Here's how the part is built. I have some questions about the finished solid (model axes, mm). A direction names the side the tool comes from. Give positions to 0.01 mm unless a question says otherwise; leave off trailing zeros. Write each loop counter-clockwise with the first axis right and the second up, starting at its lowest first coordinate (ties: lowest second). Pieces come first, ordered by that corner, then holes. Notation, with made-up numbers: (-4.5, -18.5) - (30.5, -18.5) arc R21 ccw to (30.5, 3.5) - close; hole circle Ø7 at (50, 42.25). An arc over 180 degrees is marked (long way). Use a Markdown table: item, result.
```python
from build123d import *

# Parameters (mm, degrees)
BOSS_EXTRUDE1_DEPTH    = 3
SKETCH2_R              = 1.625
CUT_EXTRUDE1_DEPTH     = 13.854960132
SKETCH3_R              = 1.625
CUT_EXTRUDE2_DEPTH     = 16.215124055
CONVERT_SOLID1_START   = -3
CONVERT_SOLID1_DEPTH   = 6
CONVERT_SOLID1_2_DEPTH = 6


# Read off the part's stored shape, not the designer's step: Convert-Solid1
with BuildPart() as part:
    # Sketch1 → Boss-Extrude1 (new, symmetric)
    with BuildSketch(Plane(origin=(0, 0, 0), x_dir=(0, 0, -1), z_dir=(1, 0, 0))):
        Polygon((0, 3.5), (0, 0), (9, 0), (9, 1.5), (1.5, 1.5), (1.5, 5), (-13.5, 5), (-13.5, 3.5), align=None)
    extrude(amount=BOSS_EXTRUDE1_DEPTH, both=True)

    # Sketch2 → Cut-Extrude1 (cut, through all)
    with BuildSketch(Plane(origin=(0, 1.5, 1.5), x_dir=(1, 0, 0), z_dir=(0, 1, 0))):
        with Locations(Location((0, 6.5, 0), (0, 0, 270))):
            Circle(SKETCH2_R)
    extrude(amount=-CUT_EXTRUDE1_DEPTH, mode=Mode.SUBTRACT)

    # Sketch3 → Cut-Extrude2 (cut, through all)
    with BuildSketch(Plane(origin=(0, 3.5, -1), x_dir=(1, 0, 0), z_dir=(0, -1, 0))):
        with Locations(Location((0, 10, 0), (0, 0, 270))):
            Circle(SKETCH3_R)
    extrude(amount=-CUT_EXTRUDE2_DEPTH, mode=Mode.SUBTRACT)

    # Convert-Solid1 outline → Convert-Solid1 (cut)
    with BuildSketch(Plane.YZ.offset(CONVERT_SOLID1_START)):
        with BuildLine():
            ThreePointArc((0, -2.25), (0.659009742, -0.659009742), (2.25, 0))
            Line((2.25, 0), (0, 0))
            Line((0, 0), (0, -2.25))
        make_face()
        with BuildLine():
            ThreePointArc((5, 0.75), (4.340990258, -0.840990258), (2.75, -1.5))
            Line((2.75, -1.5), (5, -1.5))
            Line((5, -1.5), (5, 0.75))
        make_face()
    extrude(amount=CONVERT_SOLID1_DEPTH, mode=Mode.SUBTRACT)

    # Convert-Solid1 2 outline → Convert-Solid1 2 (add)
    with BuildSketch(Plane.YZ.offset(CONVERT_SOLID1_START)):
        with BuildLine():
            ThreePointArc((3.5, 0.75), (3.280330086, 0.219669914), (2.75, 0))
            Line((2.75, 0), (3.5, 0))
            Line((3.5, 0), (3.5, 0.75))
        make_face()
        with BuildLine():
            ThreePointArc((1.5, -2.25), (1.719669914, -1.719669914), (2.25, -1.5))
            Line((2.25, -1.5), (1.5, -1.5))
            Line((1.5, -1.5), (1.5, -2.25))
        make_face()
    extrude(amount=CONVERT_SOLID1_2_DEPTH)


solid = part.part
```
Item 1: For faces 1 (the flat face through (0, 3.5, 7)), 2 (the flat face through (0, 4, 13.5)), 3 (the flat face through (0, 1.5, -7)), which set-ups out of +Z, -Z, +X, -X, +Y, -Y let a thin tool reach every point of the face, with its end or its side?
Values:
| item | result |
|---|---|
| face 1 | +Z, +X, -X, -Y |
| face 2 | +Z, +X, -X, +Y, -Y |
| face 3 | -Z, +X, -X, +Y |
Item 2: I need wall thicknesses on line 1 along Y through (x, z) = (1.9, 9); line 2 along X through (y, z) = (4.35, 9) (3 decimals); line 3 along Y through (x, z) = (1.5, -7.75). Which ranges of each line are inside material? Lowest first, please. Write a range as [from, to].
Values:
| item | result |
|---|---|
| line 1 | y = [3.5, 5] |
| line 2 | x = [-3, -1.625], [1.625, 3] |
| line 3 | y = [0, 1.5] |
Item 3: Thinking about a two-plate mould opening in X: for faces 4 (the cylindrical face through (0.071, 4.24, 10.623)), 5 (the flat face through (-3, 4, 2)), 6 (the flat face through (0, 0, -7)), which applies, +X half, -X half, draft (parallel to the pull), parting line (faces both ways), or undercut?
Values:
| item | result |
|---|---|
| face 4 | undercut |
| face 5 | -X half |
| face 6 | draft |
Item 4: If we section it at B-B, the plane x = 0: Write out the boundary of the cut face in (y, z) (3 decimals), plus the area to 3 significant figures.
Values:
| item | result |
|---|---|
| outline | (0, -9) - (1.5, -9) - (1.5, -6.625) - (0, -6.625) - close; (0, -3.375) - (1.5, -3.375) - (1.5, -2.25) arc R0.75 cw to (2.25, -1.5) - (2.75, -1.5) arc R2.25 ccw to (5, 0.75) - (5, 7.375) - (3.5, 7.375) - (3.5, 0.75) arc R0.75 cw to (2.75, 0) - (2.25, 0) arc R2.25 ccw to (0, -2.25) - close; (3.5, 10.625) - (5, 10.625) - (5, 13.5) - (3.5, 13.5) - close |
| area | 27.3 mm2 |
Item 5: If we section it at C-C, the plane y = 4.1: Write out the boundary of the cut face in (x, z) (3 decimals), plus the area to 3 significant figures.
Values:
| item | result |
|---|---|
| outline | (-3, -1.05) - (3, -1.05) - (3, 13.5) - (-3, 13.5) - close; hole circle Ø3.25 at (0, 9) |
| area | 79.0 mm2 |
Item 6: Will these pins go through, and if not, where does the flat tip stop? pin 1 Ø0.6 at (x, y) = (-0.5, 2.5) entering from -Z; pin 2 Ø3.5 at (x, z) = (0, -5) entering from -Y; pin 3 Ø1.9 at (x, z) = (0, 9) entering from +Y; pin 4 Ø3 at (x, z) = (-0.5, 9) entering from -Y.
Values:
| item | result |
|---|---|
| pin 1 | stops at z = -1.5 |
| pin 2 | stops at y = 0 |
| pin 3 | passes through |
| pin 4 | stops at y = 3.5 |
Item 7: If we section it at A-A, the plane z = -5: Write out the boundary of the cut face in (x, y) (3 decimals).
Values:
| item | result |
|---|---|
| outline | (-3, 0) - (-1.625, 0) - (-1.625, 1.5) - (-3, 1.5) - close; (1.625, 0) - (3, 0) - (3, 1.5) - (1.625, 1.5) - close |
Item 8: If we section it at D-D, the plane x = 2.2: Write out the boundary of the cut face in (y, z), plus the area to 3 significant figures.
Values:
| item | result |
|---|---|
| outline | (0, -9) - (1.5, -9) - (1.5, -2.25) arc R0.75 cw to (2.25, -1.5) - (2.75, -1.5) arc R2.25 ccw to (5, 0.75) - (5, 13.5) - (3.5, 13.5) - (3.5, 0.75) arc R0.75 cw to (2.75, 0) - (2.25, 0) arc R2.25 ccw to (0, -2.25) - close |
| area | 37.1 mm2 |
